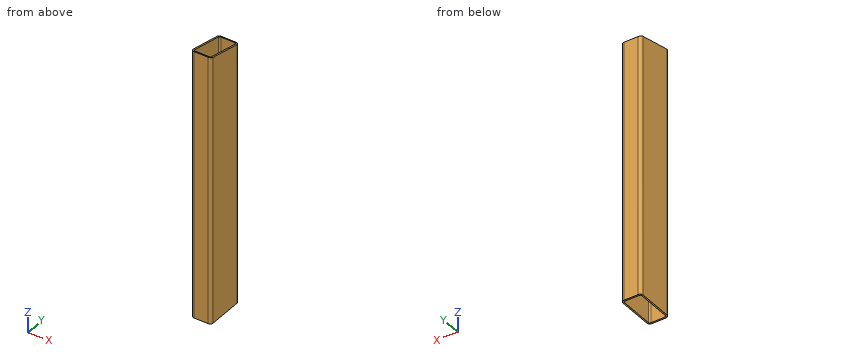
Autodesk Inventor part; units mm, degrees
ref_plane "Start Plane" through (0, 0, 80) normal (0, 0, 1) x (1, 0, 0)
ref_plane "End Plane" through (0, 0, 609.949) normal (0, 0, 1) x (1, 0, 0)
ref_plane "Work Plane4" through (14, 1823.6837, 221.6816) normal (0, 0.2039543, 0.9789804) x (1, 0, 0)
ref_plane "Start Plane" through (0, 0, 80) normal (0, 0, 1) x (1, 0, 0)
ref_plane "End Plane" through (0, 0, 609.949) normal (0, 0, 1) x (1, 0, 0)
sketch "Sketch" plane through (0, 0, 0) normal (0, 0, 1) x (1, 0, 0)
  line L0 (-20, -34) -> (-20, 34)
  line L1 (-14, 40) -> (14, 40)
  line L2 (20, 34) -> (20, -34)
  line L3 (14, -40) -> (-14, -40)
  arc A0 (-20, -34) -> (-14, -40) centre (-14, -34) ccw
  arc A1 (20, 34) -> (14, 40) centre (14, 34) ccw
  arc A2 (-14, 40) -> (-20, 34) centre (-14, 34) ccw
  arc A3 (14, -40) -> (20, -34) centre (14, -34) ccw
  arc A4 (-14, 37) -> (-17, 34) centre (-14, 34) ccw
  line L4 (-14, 37) -> (14, 37)
  arc A5 (17, 34) -> (14, 37) centre (14, 34) ccw
  line L5 (17, 34) -> (17, -34)
  arc A6 (14, -37) -> (17, -34) centre (14, -34) ccw
  line L6 (14, -37) -> (-14, -37)
  arc A7 (-17, -34) -> (-14, -37) centre (-14, -34) ccw
  line L7 (-17, -34) -> (-17, 34)
  line L8 (0, 57.7397) -> (0, -57.7397) construction
  line L9 (-29.7397, 0) -> (29.7397, 0) construction
  dimension "d7" = 6
  dimension "d9" = 40
  dimension "d11" = 80
  dimension "d12" = 3
  dimension "d15" = 20
  dimension "d16" = 40
extrude "Body" add sketch "Sketch" along normal up to surface (529.949 mm away) from surface at 80
sketch "Sketch3" plane through (0, 0, 0) normal (0, 0, 1) x (1, 0, 0)
  line L0 (0, 0) -> (10, 0)
ref_plane "Work Plane3" through (0, 0, 0) normal (0, -1, 0) x (1, 0, 0)
ref_plane "Work Plane4" through (14, 1823.6837, 221.6816) normal (0, 0.2039543, 0.9789804) x (1, 0, 0)
split "Split1" plane through (14, 1823.6837, 221.6816) removes the side toward (0, 0.2039543, 0.9789804)
sketch "Sketch4" plane through (0, 0, 0) normal (0, -1, 0) x (1, 0, 0)
  line L0 (-2, 80) -> (12, 80)
  line L1 (-2, 609.949) -> (12, 609.949)
  dimension "d18" = 529.949
equation "\"d7\" = G_IR"
equation "\"d9\" = G_W"
equation "\"d11\" = G_H"
equation "\"d12\" = G_T"
equation "\"d15\" = 0.5 * d9"
equation "\"d16\" = 0.5 * d11"
equation "\"d3\" = G_L"
equation "\"G_W\" = 40"
equation "\"G_H\" = 80"
equation "\"G_T\" = 3"
equation "\"G_IR\" = 6"
equation "\"G_L\" = d18"
equation "\"G_OFFSET_END\" = -65.051"
equation "\"d14\" = G_OFFSET_END + B_L"
equation "\"B_L\" = 675"
properties part number "ISO 10799-2 - 80x40x3 - 529.95" material "Steel, Mild"
Could you check a few things on this model? Use its own coordinates, in mm. Round coordinates to 2 decimals unless told otherwise and drop trailing zeros. Write each loop counter-clockwise with the first axis right and the second up, starting at its lowest first coordinate (ties: lowest second). Pieces come first, ordered by that corner, then holes. Notation, with made-up numbers: M -17,69.25 L 24,69.25 A20 cw 24,79.25 Z; hole C 48.25,-29 d5. An arc over 180 degrees is marked long. Answer in a Markdown table with one row per item. Add a question column.
Q1. Imagine slicing it at B-B (y = 0). Please give me the cut outline in (x, z).
Q2. Imagine slicing it at C-C (z = 496). Please give me the cut outline in (x, y), then the cut area to 3 significant figures.
Q3. Imagine slicing it at A-A (x = 3). Please give me the cut outline in (y, z).
Q4. If I drill on line 1 (Y direction, x = -10.5, z = 160.5); line 2 (X direction, y = 12.5, z = 324); line 3 (Y direction, x = -16.5, z = 502), over which ranges is the centre line in solid material (lowest first)? Write a range as from..to.
Values:
| question | item | result |
|---|---|---|
| 1 | outline | M -20,80 L -17,80 L -17,601.62 L -20,601.62 Z; M 17,80 L 20,80 L 20,601.62 L 17,601.62 Z |
| 2 | outline | M -20,-34 A6 ccw -14,-40 L 14,-40 A6 ccw 20,-34 L 20,34 A6 ccw 14,40 L -14,40 A6 ccw -20,34 Z; hole M -17,-34 A3 ccw -14,-37 L 14,-37 A3 ccw 17,-34 L 17,34 A3 ccw 14,37 L -14,37 A3 ccw -17,34 Z |
| 2 | area | 661 mm^2 |
| 3 | outline | M -40,80 L -37,80 L -37,609.32 L -40,609.95 Z; M 37,80 L 40,80 L 40,593.28 L 37,593.91 Z |
| 4 | line 1 | -40..-37, 37..40 |
| 4 | line 2 | -20..-17, 17..20 |
| 4 | line 3 | -39.45..-35.66, 35.66..39.45 |
